Source: CAD feature listing. Evaluate the final solid. Frame: model axes, mm. A direction names the side the tool comes from. Coordinates: 2 decimals unless noted, no trailing zeros. Loops run counter-clockwise (first coordinate to the right, second up) from the corner with the lowest first, then second, coordinate; pieces in that order, holes last. Notation, with made-up numbers: M -18.5,32 L 5.5,32 A21 cw 5.5,58 Z; hole C 44,-9.75 d10. An arc over 180 degrees is marked long. One line per question, with ' | ' between items. Start each with the question number.
1. Section query C-C, the plane y = -8. Output: boundary loops of the cut face in (x, z), and give its area (3 significant figures).
2. Access query for faces 4 (the flat face through (-12, 5, 0)), 5 (the flat face through (2, 7, -12)), 6 (the flat face through (2, 7, 12)), 7 (the cylindrical face through (3.35, -6.9, -6.43)). Directions: +Z, -Z, +X, -X, +Y, -Y. A direction counts if a zero-diameter tool reaches every point of the face in a straight line with its end or side. Return the directions, or none.
3. Ray query, probe 1 along Z at (x, y) = (0, 6); probe 2 along Z at (x, y) = (0, 14.5); probe 3 along X at (y, z) = (10, -0.25). Return the intervals inside material, ascending.
4. Section query A-A, the plane x = 0. Output: boundary loops of the cut face in (y, z).
5. Section query D-D, the plane z = 6.5. Output: boundary loops of the cut face in (x, y).
6. Section query B-B, the plane z = 0. Output: boundary loops of the cut face in (x, y), and give its area (3 significant figures).
7. Pin query (flat end, axial travel): P1, Ø7, axis at x = 0, z = 0, coming from the -Y side; P2, Ø2, axis at y = -4.5, z = -4, coming from the -X side; P3, Ø1, axis at y = 7.5, z = -12, coming from the +X side; P4, Ø5, axis at x = 0.5, y = -2, coming from the -Z side. Return the tip coordinate at first contact, or that it passes through.
8. Mould query, pull axis Z, two halves, no side actions, for faces 1 (the cylindrical face through (3.135, 5.773, -2.404)), 2 (the cylindrical face through (2.493, 15.14, -11.227)), 3 (the flat face through (-5.5, 0, -5.5)). Classes: pulls with the +Z half, pulls with the -Z half, needs draft (parallel to the pull), parting line crosses it, or undercut.
```python
from build123d import *

# Parameters (mm, degrees)
F0_R      = 7.25
F1_DEPTH  = 14
F3_R      = 3
F4_DEPTH  = 14.001
F6_R      = 12.75
F7_DEPTH  = 25
F8_R      = 3.95
F9_DEPTH  = 39.001
F10_R     = 12.75
F10_R_2   = 11.5
F11_DEPTH = 20
F13_DEPTH = 5


with BuildPart() as f1:
    # F0 (on Front) → F1 (new body)
    with BuildSketch(Plane.XZ):
        Circle(F0_R)
    extrude(amount=F1_DEPTH)

    # F3 (on face) → F4 (cut, through all)
    with BuildSketch(Plane.XZ.offset(14)):
        Circle(F3_R)
    extrude(amount=-F4_DEPTH, mode=Mode.SUBTRACT)

    # F6 (on offset) → F7 (join)
    with BuildSketch(Plane(origin=(0, 0, 0), x_dir=(-1, 0, 0), z_dir=(0, 1, 0))):
        Circle(F6_R)
    extrude(amount=F7_DEPTH)

    # F8 (on face) → F9 (cut, through all)
    with BuildSketch(Plane(origin=(0, 25, 0), x_dir=(-1, 0, 0), z_dir=(0, 1, 0))):
        Circle(F8_R)
    extrude(amount=-F9_DEPTH, mode=Mode.SUBTRACT)

    # F10 (on face) → F11 (cut)
    with BuildSketch(Plane(origin=(0, 25, 0), x_dir=(-1, 0, 0), z_dir=(0, 1, 0))):
        Circle(F10_R)
        Circle(F10_R_2, mode=Mode.SUBTRACT)
    extrude(amount=-F11_DEPTH, mode=Mode.SUBTRACT)

    # F12 (on face) → F13 (join)
    with BuildSketch(Plane(origin=(0, 5, 0), x_dir=(-1, 0, 0), z_dir=(0, 1, 0))):
        with BuildLine():
            ThreePointArc((2, 12.5921602595), (0, 12.75), (-2, 12.5921602595))
            Line((-2, 12.5921602595), (-2, 11.3247516529))
            ThreePointArc((-2, 11.3247516529), (0, 11.5), (2, 11.3247516529))
            Line((2, 11.3247516529), (2, 12.5921602595))
        make_face()
        with BuildLine():
            Line((-2, -11.3247516529), (-2, -12.5921602595))
            ThreePointArc((-2, -12.5921602595), (0, -12.75), (2, -12.5921602595))
            Line((2, -12.5921602595), (2, -11.3247516529))
            ThreePointArc((2, -11.3247516529), (0, -11.5), (-2, -11.3247516529))
        make_face()
    extrude(amount=F13_DEPTH)


solid = f1.part
```
Taken from the geometry:
1) outline: C 0,0 d14.5; hole C 0,0 d7.9 | area: 116 mm^2
2) face 4: -X, +Y | face 5: -Z, +X, +Y | face 6: +Z, +X, +Y | face 7: -Y
3) probe 1: -12.75 to -3.95, 3.95 to 12.75 | probe 2: -11.5 to -3.95, 3.95 to 11.5 | probe 3: -11.5 to -3.94, 3.94 to 11.5
4) outline: M -14,-7.25 L 0,-7.25 L 0,-12.75 L 10,-12.75 L 10,-11.5 L 25,-11.5 L 25,-3.95 L -14,-3.95 Z; M -14,3.95 L 25,3.95 L 25,11.5 L 10,11.5 L 10,12.75 L 0,12.75 L 0,7.25 L -14,7.25 Z
5) outline: M -10.97,0 L -3.21,0 L -3.21,-14 L 3.21,-14 L 3.21,0 L 10.97,0 L 10.97,5 L 9.49,5 L 9.49,25 L -9.49,25 L -9.49,5 L -10.97,5 Z
6) outline: M -12.75,0 L -7.25,0 L -7.25,-14 L -3.95,-14 L -3.95,25 L -11.5,25 L -11.5,5 L -12.75,5 Z; M 3.95,-14 L 7.25,-14 L 7.25,0 L 12.75,0 L 12.75,5 L 11.5,5 L 11.5,25 L 3.95,25 Z | area: 482 mm^2
7) P1: through | P2: x = -6.6 | P3: x = 2 | P4: z = -12.75
8) face 1: undercut | face 2: parting line crosses it | face 3: needs draft
